Part model, mm, in its own coordinate system. A direction names the side the tool comes from. Give positions to 0.01 mm unless a question says otherwise; leave off trailing zeros. Order: outer loops, then holes, each group sorted by start corner. A loop starts at its lowest first (then second) coordinate and runs counter-clockwise, first axis right, second up. Notation, with made-up numbers: (45, 88) - (94, 88) arc R32 ccw to (94, 120) - close; hole circle Ø6 at (68.5, 21). An arc over 180 degrees is marked (long way). Use one line per item in the form item = value. Start each with the question number.
1. Tool access for faces 1 (the face through (0, 63, 25)), 2 (the face through (4.2, -58, 26.9)), 3 (the face through (30, 61, -17)), 4 (the face through (-0.42, 70.034, -23.588)): list every direction of +Z, -Z, +X, -X, +Y, -Y with a clear straight run to the whole face (end or side of a thin tool).
2. Band-saw the part on C-C, the plane x = -52.5. List the corners of the cut face in (y, z), plus the area to 3 significant figures.
3. Band-saw the part on B-B, the plane y = -2.5. List the corners of the cut face in (x, z), plus the area to 3 significant figures.
4. Pull direction Y, two halves, no side cores. Call faces 5 (the face through (-13.65, 64.81, -29.74)), 6 (the face through (-30, 65, -15.3)), 7 (the face through (-0.42, 59.55, -35.43)): +Y half, -Y half, draft (parallel to the pull), parting line (faces both ways), or undercut.
5. Pin check, flat tips, straight feed: P1, Ø23, axis at y = 61, z = 0, coming from the +X side; P2, Ø8, axis at x = 9.5, z = -32, coming from the +Y side; P3, Ø1.5, axis at x = 32.5, z = 3, coming from the +Y side. Stop position of each tip, or through.
6. Drill centre lines: line 1 (X direction, y = 0, z = 15); line 2 (Y direction, x = 0, z = 28.3); line 3 (Z direction, x = -22.5, y = -55). Where is each one in solid material? Low to high.
7. Band-saw the part on A-A, the plane x = 0. List the corners of the cut face in (y, z), plus the area to 3 significant figures.
from build123d import *

# Parameters (mm, degrees)
SKETCH1_R                  = 63
SKETCH1_R_2                = 58
BOSS_EXTRUDE1_DEPTH        = 29.4
SKETCH2_R                  = 60.5
SKETCH2_R_2                = 58
CUT_EXTRUDE1_DEPTH         = 2
BOSS_EXTRUDE2_REACH        = 115.821
BOSS_EXTRUDE2_START_RADIUS = 63
BOSS_EXTRUDE2_END_RADIUS   = 63
SKETCH3_W                  = 60
SKETCH3_H                  = 29.4
SKETCH5_W                  = 29.4
SKETCH5_H                  = 24.463774017
CUT_EXTRUDE2_DEPTH         = 60
BOSS_EXTRUDE3_DEPTH        = 60
SKETCH7_W                  = 60
SKETCH7_H                  = 58.8
BOSS_EXTRUDE4_DEPTH        = 50
CUT_EXTRUDE3_REACH         = 184.817
SKETCH9_W                  = 60
SKETCH9_H                  = 50
BOSS_EXTRUDE5_DEPTH        = 31.44
SKETCH10_W                 = 60
SKETCH10_H                 = 31.44
BOSS_EXTRUDE6_DEPTH        = 30
SKETCH11_R                 = 58
CUT_EXTRUDE4_DEPTH         = 167.216683318
SKETCH14_W                 = 60
SKETCH14_H                 = 50.574659949
CUT_EXTRUDE5_DEPTH         = 14.7
CUT_EXTRUDE6_REACH         = 169.252
BOSS_EXTRUDE7_REACH        = 150.201
BOSS_EXTRUDE10_DEPTH       = 60
SKETCH17_R                 = 58
CUT_EXTRUDE7_DEPTH         = 148.031754667
CUT_EXTRUDE7_DEPTH_BACK    = 148.031754667
CUT_EXTRUDE13_START        = -2.5
SKETCH26_R                 = 60.5
SKETCH26_R_2               = 57.5
CUT_EXTRUDE13_DEPTH        = 10
SKETCH27_R                 = 63
SKETCH27_R_2               = 60.5
CUT_EXTRUDE14_DEPTH        = 10
SKETCH28_R                 = 82.177963531
CUT_EXTRUDE15_DEPTH        = 10
SKETCH18_W                 = 60
SKETCH18_H                 = 15
CUT_EXTRUDE8_DEPTH         = 50
SKETCH29_R                 = 2
CUT_EXTRUDE16_DEPTH        = 15
CUT_EXTRUDE17_REACH        = 150.403
SKETCH30_W                 = 60
SKETCH30_H                 = 15


with BuildPart() as part:
    # Sketch1 → Boss-Extrude1 (new body)
    with BuildSketch(Plane.XY):
        Circle(SKETCH1_R)
        Circle(SKETCH1_R_2, mode=Mode.SUBTRACT)
    extrude(amount=BOSS_EXTRUDE1_DEPTH)

    # Sketch2 → Cut-Extrude1 (cut)
    with BuildSketch(Plane.XY.offset(29.4)):
        Circle(SKETCH2_R)
        Circle(SKETCH2_R_2, mode=Mode.SUBTRACT)
    extrude(amount=-CUT_EXTRUDE1_DEPTH, mode=Mode.SUBTRACT)

    # Boss-Extrude2: from a cylinder face, 115.821 long prism both ways, kept between that surface and its translate by the depth
    boss_extrude2_start = Plane(origin=(0, 0, 14.7), z_dir=(0, 0, -1)) * Cylinder(BOSS_EXTRUDE2_START_RADIUS, 358.642, mode=Mode.PRIVATE)
    boss_extrude2_end = Plane(origin=(0, 20, 14.7), z_dir=(0, 0, -1)) * Cylinder(BOSS_EXTRUDE2_END_RADIUS, 358.642, mode=Mode.PRIVATE)
    # Sketch3 → Boss-Extrude2 (add, from a surface)
    with BuildSketch(Plane(origin=(0, 0, 0), x_dir=(1, 0, 0), z_dir=(0, 1, 0)), mode=Mode.PRIVATE) as boss_extrude2_sk1:
        with Locations((0, -14.7)):
            Rectangle(SKETCH3_W, SKETCH3_H)
    boss_extrude2_tool1 = extrude(boss_extrude2_sk1.sketch, amount=BOSS_EXTRUDE2_REACH, both=True, mode=Mode.PRIVATE)
    add(((boss_extrude2_tool1 - boss_extrude2_start) & boss_extrude2_end).solids().sort_by_distance((0, 65.398556, 14.7))[0])

    # Sketch5 → Cut-Extrude2 (cut)
    with BuildSketch(Plane.ZY.offset(30)):
        with Locations((14.7, 87.630442947)):
            Rectangle(SKETCH5_W, SKETCH5_H)
    extrude(amount=-CUT_EXTRUDE2_DEPTH, mode=Mode.SUBTRACT)

    # Sketch6 → Boss-Extrude3 (add)
    with BuildSketch(Plane.ZY.offset(30)):
        Polygon((0, 75.398555938), (29.4, 126.32084968), (29.4, 75.398555938), align=None)
    extrude(amount=-BOSS_EXTRUDE3_DEPTH)

    # Sketch7 → Boss-Extrude4 (add)
    with BuildSketch(Plane(origin=(0, 18.849638984, -32.648532425), x_dir=(1, 0, 0), z_dir=(0, 0.500000000000004, -0.8660254037844364))):
        with Locations((0, -94.697064851)):
            Rectangle(SKETCH7_W, SKETCH7_H)
    extrude(amount=BOSS_EXTRUDE4_DEPTH)

    # Sketch8 → Cut-Extrude3 (cut, up to next)
    with BuildSketch(Plane(origin=(30, 0, 0), x_dir=(0, 0, -1), z_dir=(1, 0, 0)), mode=Mode.PRIVATE) as cut_extrude3_sk1:
        Polygon((28.601270189, 125.859702809), (-29.4, 92.372653852), (-29.4, 126.32084968), (13.901270189, 151.32084968), align=None)
    cut_extrude3_tool1 = extrude(cut_extrude3_sk1.sketch, amount=-CUT_EXTRUDE3_REACH, mode=Mode.PRIVATE) & part.part
    add(cut_extrude3_tool1.solids().sort_by_distance((30, 123.250107, 3.896605))[0], mode=Mode.SUBTRACT)

    # Sketch9 → Boss-Extrude5 (add)
    with BuildSketch(Plane(origin=(0, 56.548916953, 32.648532425), x_dir=(1, 0, 0), z_dir=(0, -0.8660254037844365, -0.500000000000004))):
        with Locations((0, -62.699277969)):
            Rectangle(SKETCH9_W, SKETCH9_H)
    extrude(amount=BOSS_EXTRUDE5_DEPTH)

    # Sketch10 → Boss-Extrude6 (add)
    with BuildSketch(Plane(origin=(0, 18.849638984, -32.648532425), x_dir=(1, 0, 0), z_dir=(0, -0.500000000000004, 0.8660254037844364))):
        with Locations((0, 49.577064851)):
            Rectangle(SKETCH10_W, SKETCH10_H)
    extrude(amount=BOSS_EXTRUDE6_DEPTH)

    # Sketch11 → Cut-Extrude4 (cut, through all)
    with BuildSketch(Plane.XY.offset(29.4)):
        with Locations(Location((0, 0, 0), (0, 0, 121.147389922))):
            Circle(SKETCH11_R)
    extrude(amount=-CUT_EXTRUDE4_DEPTH, mode=Mode.SUBTRACT)

    # Sketch14 → Cut-Extrude5 (cut)
    with BuildSketch(Plane.XY.offset(29.4)):
        with Locations((0, 117.659983826)):
            Rectangle(SKETCH14_W, SKETCH14_H)
        with BuildLine():
            ThreePointArc((30, 55.398555938), (0, 63), (-30, 55.398555938))
            Line((-30, 55.398555938), (-30, 92.372653852))
            Line((-30, 92.372653852), (30, 92.372653852))
            Line((30, 92.372653852), (30, 55.398555938))
        make_face()
    extrude(amount=-CUT_EXTRUDE5_DEPTH, mode=Mode.SUBTRACT)

    # Sketch15 → Cut-Extrude6 (cut, up to next)
    with BuildSketch(Plane(origin=(30, 0, 0), x_dir=(0, 0, -1), z_dir=(1, 0, 0)), mode=Mode.PRIVATE) as cut_extrude6_sk1:
        Polygon((44.021270189, 99.151479356), (-14.7, 65.248738206), (-14.7, 100.859702809), (28.601270189, 125.859702809), align=None)
    cut_extrude6_tool1 = extrude(cut_extrude6_sk1.sketch, amount=-CUT_EXTRUDE6_REACH, mode=Mode.PRIVATE) & part.part
    add(cut_extrude6_tool1.solids().sort_by_distance((30, 96.99498, -10.999854))[0], mode=Mode.SUBTRACT)

    # Boss-Extrude7: up to this face of the body (flat: up to its plane)
    boss_extrude7_end = Plane(part.part.faces().sort_by_distance((-30, 70.930733499, -23.393070455))[0])
    # Sketch16 → Boss-Extrude7 (add, up to the picked face)
    with BuildSketch(Plane(origin=(30, 0, 0), x_dir=(0, 0, -1), z_dir=(1, 0, 0)), mode=Mode.PRIVATE) as boss_extrude7_sk1:
        Polygon((-17.904609691, 55.398555938), (-14.7, 55.398555938), (-14.7, 65.248738206), (-17.904609691, 63.398555938), align=None)
    boss_extrude7_tool1 = split(extrude(boss_extrude7_sk1.sketch, amount=-BOSS_EXTRUDE7_REACH, mode=Mode.PRIVATE), bisect_by=boss_extrude7_end, keep=Keep.BOTH, mode=Mode.PRIVATE)
    add(boss_extrude7_tool1.solids().sort_by(Axis((30, 59.877083, 16.246945), (-1, 0, 0)))[0])

    # Sketch25 → Boss-Extrude10 (add)
    with BuildSketch(Plane(origin=(30, 0, 0), x_dir=(0, 0, -1), z_dir=(1, 0, 0))):
        Polygon((-17.904609691, 55.398555938), (-31.761016151, 55.398555938), (-17.904609691, 63.398555938), align=None)
    extrude(amount=-BOSS_EXTRUDE10_DEPTH)

    # Sketch17 → Cut-Extrude7 (cut, two sides)
    with BuildSketch(Plane.XY.offset(29.4)) as cut_extrude7_sk:
        with Locations(Location((0, 0, 0), (0, 0, 121.147389922))):
            Circle(SKETCH17_R)
    extrude(amount=CUT_EXTRUDE7_DEPTH, mode=Mode.SUBTRACT)
    extrude(cut_extrude7_sk.sketch, amount=-CUT_EXTRUDE7_DEPTH_BACK, mode=Mode.SUBTRACT)

    # Sketch26 → Cut-Extrude13 (cut)
    with BuildSketch(Plane.XY.offset(29.4).offset(CUT_EXTRUDE13_START)):
        Circle(SKETCH26_R)
        Circle(SKETCH26_R_2, mode=Mode.SUBTRACT)
    extrude(amount=CUT_EXTRUDE13_DEPTH, mode=Mode.SUBTRACT)

    # Sketch27 → Cut-Extrude14 (cut)
    with BuildSketch(Plane.XY.offset(29.4)):
        Circle(SKETCH27_R)
        Circle(SKETCH27_R_2, mode=Mode.SUBTRACT)
    extrude(amount=CUT_EXTRUDE14_DEPTH, mode=Mode.SUBTRACT)

    # Sketch28 → Cut-Extrude15 (cut)
    with BuildSketch(Plane.XY.offset(29.4)):
        Circle(SKETCH28_R)
    extrude(amount=CUT_EXTRUDE15_DEPTH, mode=Mode.SUBTRACT)

    # Sketch18 → Cut-Extrude8 (cut)
    with BuildSketch(Plane(origin=(0, 43.849638984, -75.949802615), x_dir=(1, 0, 0), z_dir=(0, 0.500000000000004, -0.8660254037844364))):
        with Locations((0, -56.357064851)):
            Rectangle(SKETCH18_W, SKETCH18_H)
    extrude(amount=-CUT_EXTRUDE8_DEPTH, mode=Mode.SUBTRACT)

    # Sketch29 → Cut-Extrude16 (cut)
    with BuildSketch(Plane(origin=(0, 29.321078258, 16.928532425), x_dir=(1, 0, 0), z_dir=(0, -0.8660254037844362, -0.5000000000000041))):
        with Locations(Location((-15, -59.636899675, 0), (0, 0, 270))):
            Circle(SKETCH29_R)
        with Locations(Location((15, -59.636899675, 0), (0, 0, 270))):
            Circle(SKETCH29_R)
    extrude(amount=-CUT_EXTRUDE16_DEPTH, mode=Mode.SUBTRACT)

    # Sketch30 → Cut-Extrude17 (cut, up to next)
    with BuildSketch(Plane(origin=(0, 42.311459315, 24.428532425), x_dir=(1, 0, 0), z_dir=(0, 0.8660254037844364, 0.5000000000000041)), mode=Mode.PRIVATE) as cut_extrude17_sk1:
        with Locations((0, 80.199277969)):
            Rectangle(SKETCH30_W, SKETCH30_H)
    cut_extrude17_tool1 = extrude(cut_extrude17_sk1.sketch, amount=-CUT_EXTRUDE17_REACH, mode=Mode.PRIVATE) & part.part
    add(cut_extrude17_tool1.solids().sort_by_distance((0, 82.411098, -45.02608))[0], mode=Mode.SUBTRACT)


solid = part.part
From the geometry:
q1.face_1 = +Z, +Y
q1.face_2 = +Z
q1.face_3 = -Z, +X, +Y
q1.face_4 = +X, -X, +Y
q2.outline = (-34.82, 0) - (-24.65, 0) - (-24.65, 26.9) - (-30.07, 26.9) - (-30.07, 29.4) - (-34.82, 29.4) - close; (24.65, 0) - (34.82, 0) - (34.82, 29.4) - (30.07, 29.4) - (30.07, 26.9) - (24.65, 26.9) - close
q2.area = 571 mm²
q3.outline = (-62.95, 0) - (-57.95, 0) - (-57.95, 26.9) - (-60.45, 26.9) - (-60.45, 29.4) - (-62.95, 29.4) - close; (57.95, 0) - (62.95, 0) - (62.95, 29.4) - (60.45, 29.4) - (60.45, 26.9) - (57.95, 26.9) - close
q3.area = 282 mm²
q4.face_5 = undercut
q4.face_6 = draft
q4.face_7 = -Y half
q5.P1 = 38.97
q5.P2 = 77.2
q5.P3 = 54.41
q6.line_1 = -63 to -58, 58 to 63
q6.line_2 = -63 to -60.5, 60.5 to 63
q6.line_3 = 0 to 26.9
q7.outline = (-63, 0) - (-58, 0) - (-58, 26.9) - (-60.5, 26.9) - (-60.5, 29.4) - (-63, 29.4) - close; (58, -32.74) - (65.67, -46.03) - (78.66, -38.53) - (61.16, -8.22) - (74.15, -0.72) - (63, 18.59) - (63, 29.4) - (60.5, 29.4) - (60.5, 26.9) - (58, 26.9) - close
q7.area = 882 mm²
